Part model, mm, in its own coordinate system. A direction names the side the tool comes from. Round coordinates to 2 decimals unless told otherwise and drop trailing zeros. Order: outer loops, then holes, each group sorted by start corner. A loop starts at its lowest first (then second) coordinate and runs counter-clockwise, first axis right, second up. Notation, with made-up numbers: (86, 44.5) - (132, 44.5) arc R24 cw to (132, 81.5) - close; hole circle Ø11 at (32, 17). An arc over 180 degrees is marked (long way). Return JSON: item names as keys, results as strings. Group by question number.
Item 1: Tool access for faces 1 (the face through (-3.045, 2.335, 225.374)), 2 (the face through (5.96, -1.88, 56.7)): list every direction of +Z, -Z, +X, -X, +Y, -Y with a clear straight run to the whole face (end or side of a thin tool).
Item 2: Drop flat-ended pins along their axis: pin 1 (5 mm diameter, centred on x = 3.5, z = 186.5, fed in from +Y); pin 2 (8 mm diameter, centred on y = 1, z = 102.5, fed in from +X); pin 3 (1 mm diameter, centred on x = 3, z = 98.5, fed in from +Y). Give the stop position or say it passes through.
Item 3: Probe probe 1 along Y at (x, z) = (0, 116); probe 2 along Y at (x, z) = (5.5, 120); probe 3 along X at (y, z) = (-2.25, 208.5). List the from-to ranges inside material, lowest first.
Item 4: Saw through at A-A on z = 125. List the corners of the cut face in (x, y).
Item 5: Saw through at B-B on z = 23. List the corners of the cut face in (x, y), and give its area (3 significant figures).
Autodesk Inventor part; units mm, degrees
ref_plane "YZ Plane" through (0, 0, 0) normal (1, 0, 0) x (0, 1, 0)
ref_plane "XZ Plane" through (0, 0, 0) normal (0, 1, 0) x (-1, 0, 0)
ref_plane "XY Plane" through (0, 0, 0) normal (0, 0, 1) x (1, 0, 0)
sketch "スケッチ5" plane through (0, 0, 0) normal (0, 0, 1) x (1, 0, 0)
  circle A0 centre (0, 0) radius 6.25
  dimension "d14" = 12.5
extrude "押し出し5" add sketch "スケッチ5" along normal blind 115
sketch "スケッチ6" plane through (0, 0, 115) normal (0, 0, 1) x (1, 0, 0)
  circle A0 centre (0, 0) radius 6.35
  dimension "d17" = 12.7
extrude "押し出し6" add sketch "スケッチ6" along normal blind 50
sketch "スケッチ7" plane through (0, 0, 165) normal (0, 0, 1) x (1, 0, 0)
  circle A0 centre (0, 0) radius 6.25
  dimension "d20" = 12.5
extrude "押し出し7" add sketch "スケッチ7" along normal blind 29
sketch "スケッチ8" plane through (0, 0, 194) normal (0, 0, 1) x (1, 0, 0)
  circle A0 centre (0, 0) radius 6.2
  dimension "d23" = 12.4
extrude "押し出し8" add sketch "スケッチ8" along normal blind 15 draft 2
sketch "スケッチ9" plane through (0, 0, 209) normal (0, 0, 1) x (1, 0, 0)
  circle A0 centre (0, 0) radius 6.7238
extrude "押し出し9" add sketch "スケッチ9" along normal blind 33 draft -10
fillet "フィレット3" radius 2 1 edges at (-6.7238, 0, 209)
properties part number "hude"
Filled in:
{
 "1": {"face 1": "+Z", "face 2": "-Z"},
 "2": {"pin 1": "stops at y = 6.17", "pin 2": "stops at x = 6.25", "pin 3": "stops at y = 5.73"},
 "3": {"probe 1": "y = -6.35 to 6.35", "probe 2": "y = -3.17 to 3.17", "probe 3": "x = -6.32 to 6.32"},
 "4": {"outline": "circle Ø12.7 at (0, 0)"},
 "5": {"outline": "circle Ø12.5 at (0, 0)", "area": "123 mm^2"}
}
